```python
from build123d import *

# Parameters (mm, degrees)
F4_DEPTH = 5.2
F5_R     = 2


with BuildPart() as f2:
    # F1 (on Front) → F2 (revolve)
    with BuildSketch(Plane.XZ):
        with BuildLine():
            ThreePointArc((0, 7.2088790199), (-6.1637637999, 5.2187873117), (-10, 0))
            Line((-10, 0), (0, 0))
            Line((0, 0), (0, 7.2088790199))
        make_face()
    revolve(axis=Axis((0, 0, 3.60443951), (0, 0, 1)))

    # F3 (on face) → F4 (cut)
    with BuildSketch(Plane(origin=(0, 0, 0), x_dir=(1, 0, 0), z_dir=(0, 0, -1))):
        Polygon((2.35, 4.0703193978), (-2.35, 4.0703193978), (-4.7, 0), (-2.35, -4.0703193978), (2.35, -4.0703193978), (4.7, 0), align=None)
    extrude(amount=-F4_DEPTH, mode=Mode.SUBTRACT)

    # F5
    f5_edges = [f2.edges().sort_by_distance(p)[0] for p in [
        (0, -4.070319, 5.2),
        (-3.525, -2.03516, 5.2),
        (3.525, -2.03516, 5.2),
        (3.525, 2.03516, 5.2),
        (-3.525, 2.03516, 5.2),
        (0, 4.070319, 5.2),
    ]]
    fillet(f5_edges, radius=F5_R)


solid = f2.part
```
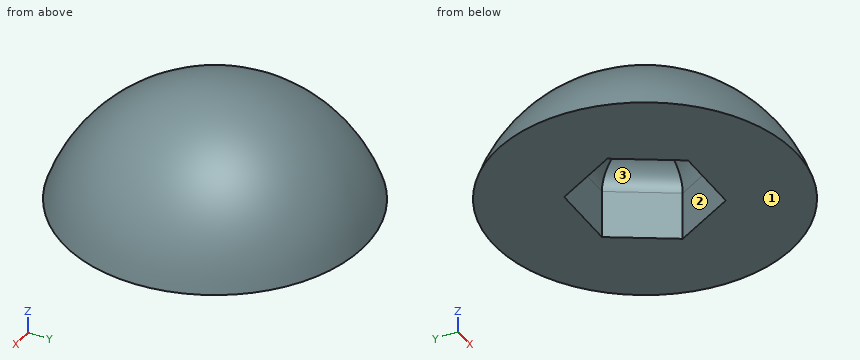
The model under review builds one solid part; all positions refer to its coordinate system, in mm. Face numbers are marked on the shaded views. Coordinates: 2 decimals unless noted, no trailing zeros. Order: outer loops, then holes, each group sorted by start corner. A loop starts at its lowest first (then second) coordinate and runs counter-clockwise, first axis right, second up. Notation, with made-up numbers: (62.25, 38.25) -> (68.25, 38.25) arc R30 ccw to (68.25, 71.25) -> close; hole circle Ø11 at (3, -29.75). An arc over 180 degrees is marked (long way). Answer in a Markdown table with one row per item. Add a question column.
Item 1: We need section A-A on z = 1.5. Write out the cut boundary in (x, y).
Item 2: Mouldability with a two-part tool opening along Y and no side actions: class the marked faces 1, 2 and 3 as +Y half, -Y half, draft (parallel to the pull), parting line (faces both ways), or undercut.
Item 3: To check wall thickness, follow probe 1 along Y at (x, z) = (1, 2.5); probe 2 along X at (y, z) = (-2, 3.5); probe 3 along Y at (x, z) = (-2.5, 2.5). State the ranges of each line that lie inside material, in increasing order.
Item 4: Clearance check with flat-ended pins moving along their axes: pin 1 (1.5 mm diameter, centred on y = -2, z = 1.5, fed in from -X); pin 2 (4.5 mm diameter, centred on x = 0.5, y = 0.5, fed in from -Z); pin 3 (1.5 mm diameter, centred on x = 5, y = -6, fed in from +Z). State where each tip first meets the part, or that it passes through.
Item 5: We need section B-B on y = 6.75. Write out the cut boundary in (x, z), plus the area to 3 significant figures.
Item 6: We need section D-D on x = 7.5. Write out the cut boundary in (y, z).
Item 7: We need section C-C on z = 2.75. Write out the cut boundary in (x, y).
Final values:
| question | item | result |
|---|---|---|
| 1 | outline | circle Ø18.74 at (0, 0); hole (-4.7, 0) -> (-2.35, -4.07) -> (2.35, -4.07) -> (4.7, 0) -> (2.35, 4.07) -> (-2.35, 4.07) -> close |
| 2 | face 1 | draft |
| 2 | face 2 | undercut |
| 2 | face 3 | undercut |
| 3 | probe 1 | y = -8.72 to -4.07, 4.07 to 8.72 |
| 3 | probe 2 | x = -7.77 to -3.52, 3.52 to 7.77 |
| 3 | probe 3 | y = -8.42 to -3.81, 3.81 to 8.42 |
| 4 | pin 1 | stops at x = -9.54 |
| 4 | pin 2 | stops at z = 5 |
| 4 | pin 3 | stops at z = 4.49 |
| 5 | outline | (-7.38, 0) -> (7.38, 0) arc R8.1 ccw to start |
| 5 | area | 50.6 mm2 |
| 6 | outline | (-6.61, 0) -> (6.61, 0) arc R7.41 ccw to start |
| 7 | outline | circle Ø17.22 at (0, 0); hole (-4.7, 0) -> (-2.35, -4.07) -> (2.35, -4.07) -> (4.7, 0) -> (2.35, 4.07) -> (-2.35, 4.07) -> close |
